from build123d import *

# Parameters (mm, degrees)
SKETCH1_W                 = 100
SKETCH1_H                 = 70
BOSS_EXTRUDE1_DEPTH       = 10
SKETCH2_R                 = 10
CUT_EXTRUDE1_DEPTH        = 11
F_3_0MM_DOWEL_HOLE1_D     = 3
F_3_0MM_DOWEL_HOLE1_DEPTH = 5
F_3_0MM_DOWEL_HOLE1_TIP   = 0.901290929
FILLET2_R                 = 15


with BuildPart() as part:
    # Sketch1 → Boss-Extrude1 (new body)
    with BuildSketch(Plane(origin=(0, 0, 0), x_dir=(1, 0, 0), z_dir=(0, 1, 0))):
        Rectangle(SKETCH1_W, SKETCH1_H)
    extrude(amount=BOSS_EXTRUDE1_DEPTH)

    # Sketch2 → Cut-Extrude1 (cut, through all)
    with BuildSketch(Plane(origin=(0, 10, 0), x_dir=(1, 0, 0), z_dir=(0, 1, 0))):
        Circle(SKETCH2_R)
    extrude(amount=-CUT_EXTRUDE1_DEPTH, mode=Mode.SUBTRACT)

    # Ø3.0mm Dowel Hole1
    with Locations(Plane(origin=(0, 0, 0), x_dir=(-1, 0, 0), z_dir=(0, -1, 0))):
        with Locations((40, 0), (-40, 0)):
            Hole(F_3_0MM_DOWEL_HOLE1_D / 2, depth=F_3_0MM_DOWEL_HOLE1_DEPTH)
            with Locations((0, 0, -(F_3_0MM_DOWEL_HOLE1_DEPTH + F_3_0MM_DOWEL_HOLE1_TIP / 2))):  # 118° drill point
                Cone(0, F_3_0MM_DOWEL_HOLE1_D / 2, F_3_0MM_DOWEL_HOLE1_TIP, mode=Mode.SUBTRACT)

    # Fillet2
    fillet2_edges = [part.edges().sort_by_distance(p)[0] for p in [
        (-50, 5, -35),
        (50, 5, -35),
        (50, 5, 35),
        (-50, 5, 35),
    ]]
    fillet(fillet2_edges, radius=FILLET2_R)


solid = part.part
The listing builds one solid part. Answer for the finished solid, in the listing's coordinates (mm). A direction names the side the tool comes from. Round coordinates to 2 decimals unless told otherwise and drop trailing zeros. Order: outer loops, then holes, each group sorted by start corner. A loop starts at its lowest first (then second) coordinate and runs counter-clockwise, first axis right, second up. Notation, with made-up numbers: (7.5, 75) - (23.5, 75) arc R7 cw to (23.5, 87) - close; hole circle Ø1 at (79.25, -10). An arc over 180 degrees is marked (long way). Write item = value, one per line. Start each with the question number.
1) Section D-D, the plane y = 2.75 is taken. Write down the section's boundary in (x, z), plus the area to 3 significant figures.
2) For faces 5 (the flat face through (10.4, 0, -0.5)), 6 (the cylindrical face through (-41.5, 2.54, -0.07)), determine the directions among +Z, -Z, +X, -X, +Y, -Y from which every point of the face is accessible in a straight line to the end or side of a thin tool.
3) Straight lines are drawn through the part: L1, parallel to Z at x = 0, y = 4; L2, parallel to Z at x = 40, y = 1.3; L3, parallel to X at y = 0.5, z = 7. For each, find the intervals that lie inside material, in ascending order.
4) Section A-A, the plane x = 0 is taken. Write down the section's boundary in (y, z).
5) Given pin 1 (1 mm diameter, centred on y = 2, z = -21.5, fed in from -X); pin 2 (2.5 mm diameter, centred on x = -40, z = 0, fed in from -Y); pin 3 (1 mm diameter, centred on y = 7.5, z = 24.5, fed in from +X); pin 4 (18 mm diameter, centred on x = 0, z = 0, fed in from +Y), each flat-ended and moving along its own axis, determine where each tip first touches the part or whether it passes through.
6) Section B-B, the plane y = 8 is taken. Write down the section's boundary in (x, z), plus the area to 3 significant figures.
7) For a pull along X with two mould halves and no side action, classify faces 1 (the cylindrical face through (-45.72, 5.07, 30.49)), 2 (the flat face through (0, 5, 35)), 3 (the conical face through (-39.808, 5.745, -0.176)), 4 (the cylindrical face through (45.49, 5.07, -30.72)) as released by +X, released by -X, zero draft, split by the parting line, or undercut.
8) Section C-C, the plane z = 6.5 is taken. Write down the section's boundary in (x, y), plus the area to 3 significant figures.
Results list:
q1.outline = (-50, -20) arc R15 ccw to (-35, -35) - (35, -35) arc R15 ccw to (50, -20) - (50, 20) arc R15 ccw to (35, 35) - (-35, 35) arc R15 ccw to (-50, 20) - close; hole circle Ø3 at (-40, 0); hole circle Ø20 at (0, 0); hole circle Ø3 at (40, 0)
q1.area = 6,480 mm^2
q2.face_5 = +Z, -Z, +X, -X, -Y
q2.face_6 = -Y
q3.L1 = -35 to -10, 10 to 35
q3.L2 = -34.14 to -1.5, 1.5 to 34.14
q3.L3 = -50 to -7.14, 7.14 to 50
q4.outline = (0, -35) - (10, -35) - (10, -10) - (0, -10) - close; (0, 10) - (10, 10) - (10, 35) - (0, 35) - close
q5.pin_1 = -49.97
q5.pin_2 = 5.15
q5.pin_3 = 49.46
q5.pin_4 = through
q6.outline = (-50, -20) arc R15 ccw to (-35, -35) - (35, -35) arc R15 ccw to (50, -20) - (50, 20) arc R15 ccw to (35, 35) - (-35, 35) arc R15 ccw to (-50, 20) - close; hole circle Ø20 at (0, 0)
q6.area = 6,490 mm^2
q7.face_1 = released by -X
q7.face_2 = zero draft
q7.face_3 = undercut
q7.face_4 = released by +X
q8.outline = (-50, 0) - (-7.6, 0) - (-7.6, 10) - (-50, 10) - close; (7.6, 0) - (50, 0) - (50, 10) - (7.6, 10) - close
q8.area = 848 mm^2
